Geometry check sheet. Reference: the model listing, model coordinates, mm. Round coordinates to 2 decimals unless told otherwise and drop trailing zeros. Loops run counter-clockwise (first coordinate to the right, second up) from the corner with the lowest first, then second, coordinate; pieces in that order, holes last. Notation, with made-up numbers: (62.25, 22.25) - (82.25, 22.25) arc R15 cw to (82.25, 36.25) - close; hole circle Ø6 at (22, 71). An arc over 180 degrees is marked (long way). Answer as CSV lines item,"result". Start each with the question number.
1) Cross-section at D-D on x = 65. Record the boundary of the cut face in (y, z).
2) Thickness scan on line 1 along X through (y, z) = (0.9, -57); line 2 along X through (y, z) = (2.25, -175); line 3 along X through (y, z) = (1.7, -333). Record the ranges inside material, lowest first.
3) Cross-section at A-A on z = -260.5. Record the boundary of the cut face in (x, y).
4) Depth check by flat-ended pin: P1, Ø2.5, axis at y = 2, z = -341.5, coming from the -X side; P2, Ø10, axis at x = 152, z = -266.5, coming from the -Y side. Enter the tip coordinate at first touch or a pass-through.
5) Cross-section at B-B on x = 34.5. Record the boundary of the cut face in (y, z), and give its area (3 significant figures).
6) Draft check along Z on faces 1 (the cylindrical face through (246.99, 2.46, -2.85)), 2 (the cylindrical face through (247.15, 2.46, -346.99)), 3 (the cylindrical face through (162.63, 2.46, -169.27)). Enter one of: released by +Z, released by -Z, zero draft, split by the parting line, or undercut.
7) Cross-section at C-C on z = -213. Record the boundary of the cut face in (x, y), and give its area (3 significant figures).
from build123d import *

# Parameters (mm, degrees)
SKETCH1_R           = 1.5
SKETCH1_W           = 30
SKETCH1_H           = 5
SKETCH1_W_2         = 5
SKETCH1_H_2         = 50
SKETCH1_R_2         = 3
SKETCH1_R_3         = 4
SKETCH1_W_3         = 60
SKETCH1_R_4         = 6.2
SKETCH1_R_5         = 9.5
SKETCH1_W_4         = 98
SKETCH1_H_3         = 41
SKETCH1_H_4         = 100
BOSS_EXTRUDE1_DEPTH = 5


with BuildPart() as part:
    # Sketch1 → Boss-Extrude1 (new body)
    # profile 1 of 2: a face of its own
    with BuildSketch(Plane(origin=(0, 0, 0), x_dir=(1, 0, 0), z_dir=(0, 1, 0))):
        with BuildLine():
            ThreePointArc((0, 10), (2.928932188, 2.928932188), (10, 0))
            Line((10, 0), (240, 0))
            ThreePointArc((240, 0), (247.071067812, 2.928932188), (250, 10))
            Line((250, 10), (250, 340))
            ThreePointArc((250, 340), (247.071067812, 347.071067812), (240, 350))
            Line((240, 350), (10, 350))
            ThreePointArc((10, 350), (2.928932188, 347.071067812), (0, 340))
            Line((0, 340), (0, 10))
        make_face()
        with Locations(Location((17, 17, 0), (0, 0, 270))):
            Circle(SKETCH1_R, mode=Mode.SUBTRACT)
        with Locations((42, 9.5)):
            Rectangle(SKETCH1_W, SKETCH1_H, mode=Mode.SUBTRACT)
        with Locations((9.5, 52)):
            Rectangle(SKETCH1_W_2, SKETCH1_H_2, mode=Mode.SUBTRACT)
        with Locations(Location((45, 147.266112644, 0), (0, 0, 270))):
            Circle(SKETCH1_R_2, mode=Mode.SUBTRACT)
        with Locations(Location((65, 125, 0), (0, 0, 270))):
            Circle(SKETCH1_R_3, mode=Mode.SUBTRACT)
        with Locations(Location((105, 125, 0), (0, 0, 270))):
            Circle(SKETCH1_R_3, mode=Mode.SUBTRACT)
        with Locations((125, 9.5)):
            Rectangle(SKETCH1_W_3, SKETCH1_H, mode=Mode.SUBTRACT)
        with Locations((208, 9.5)):
            Rectangle(SKETCH1_W, SKETCH1_H, mode=Mode.SUBTRACT)
        with Locations(Location((233, 17, 0), (0, 0, 270))):
            Circle(SKETCH1_R, mode=Mode.SUBTRACT)
        with Locations((240.5, 52)):
            Rectangle(SKETCH1_W_2, SKETCH1_H_2, mode=Mode.SUBTRACT)
        with Locations(Location((145, 125, 0), (0, 0, 270))):
            Circle(SKETCH1_R_3, mode=Mode.SUBTRACT)
        with Locations(Location((185, 125, 0), (0, 0, 270))):
            Circle(SKETCH1_R_3, mode=Mode.SUBTRACT)
        with Locations(Location((205, 147.266112644, 0), (0, 0, 270))):
            Circle(SKETCH1_R_2, mode=Mode.SUBTRACT)
        Polygon((7, 175), (7, 225), (12, 225), (12, 125), (7, 125), align=None, mode=Mode.SUBTRACT)
        with Locations(Location((17, 206, 0), (0, 0, 270))):
            Circle(SKETCH1_R, mode=Mode.SUBTRACT)
        with Locations(Location((45, 202.733887356, 0), (0, 0, 270))):
            Circle(SKETCH1_R_2, mode=Mode.SUBTRACT)
        with Locations(Location((85, 175, 0), (0, 0, 270))):
            Circle(SKETCH1_R_4, mode=Mode.SUBTRACT)
        with Locations(Location((78.5, 225.5, 0), (0, 0, 270))):
            Circle(SKETCH1_R, mode=Mode.SUBTRACT)
        with Locations((9.5, 298)):
            Rectangle(SKETCH1_W_2, SKETCH1_H_2, mode=Mode.SUBTRACT)
        with Locations(Location((17, 333, 0), (0, 0, 270))):
            Circle(SKETCH1_R, mode=Mode.SUBTRACT)
        with Locations((42, 340.5)):
            Rectangle(SKETCH1_W, SKETCH1_H, mode=Mode.SUBTRACT)
        with Locations(Location((78.5, 280.5, 0), (0, 0, 270))):
            Circle(SKETCH1_R, mode=Mode.SUBTRACT)
        with Locations(Location((125, 175, 0), (0, 0, 270))):
            Circle(SKETCH1_R_5, mode=Mode.SUBTRACT)
        with Locations(Location((165, 175, 0), (0, 0, 270))):
            Circle(SKETCH1_R_4, mode=Mode.SUBTRACT)
        with Locations((125, 253)):
            Rectangle(SKETCH1_W_4, SKETCH1_H_3, mode=Mode.SUBTRACT)
        with Locations(Location((171.5, 225.5, 0), (0, 0, 270))):
            Circle(SKETCH1_R, mode=Mode.SUBTRACT)
        with Locations(Location((205, 202.733887356, 0), (0, 0, 270))):
            Circle(SKETCH1_R_2, mode=Mode.SUBTRACT)
        with Locations((240.5, 175)):
            Rectangle(SKETCH1_W_2, SKETCH1_H_4, mode=Mode.SUBTRACT)
        with Locations(Location((233, 206, 0), (0, 0, 270))):
            Circle(SKETCH1_R, mode=Mode.SUBTRACT)
        with Locations(Location((171.5, 280.5, 0), (0, 0, 270))):
            Circle(SKETCH1_R, mode=Mode.SUBTRACT)
        Polygon((95, 343), (125, 343), (155, 343), (155, 338), (95, 338), align=None, mode=Mode.SUBTRACT)
        with Locations((240.5, 298)):
            Rectangle(SKETCH1_W_2, SKETCH1_H_2, mode=Mode.SUBTRACT)
        with Locations((208, 340.5)):
            Rectangle(SKETCH1_W, SKETCH1_H, mode=Mode.SUBTRACT)
        with Locations(Location((233, 333, 0), (0, 0, 270))):
            Circle(SKETCH1_R, mode=Mode.SUBTRACT)
    # profile 2 of 2: a face of its own
    with BuildSketch(Plane(origin=(0, 0, 0), x_dir=(1, 0, 0), z_dir=(0, 1, 0))):
        with BuildLine():
            ThreePointArc((0, 10), (2.928932188, 2.928932188), (10, 0))
            Line((10, 0), (240, 0))
            ThreePointArc((240, 0), (247.071067812, 2.928932188), (250, 10))
            Line((250, 10), (250, 340))
            ThreePointArc((250, 340), (247.071067812, 347.071067812), (240, 350))
            Line((240, 350), (10, 350))
            ThreePointArc((10, 350), (2.928932188, 347.071067812), (0, 340))
            Line((0, 340), (0, 10))
        make_face()
        with Locations(Location((17, 17, 0), (0, 0, 270))):
            Circle(SKETCH1_R, mode=Mode.SUBTRACT)
        with Locations((42, 9.5)):
            Rectangle(SKETCH1_W, SKETCH1_H, mode=Mode.SUBTRACT)
        with Locations((9.5, 52)):
            Rectangle(SKETCH1_W_2, SKETCH1_H_2, mode=Mode.SUBTRACT)
        with Locations(Location((45, 147.266112644, 0), (0, 0, 270))):
            Circle(SKETCH1_R_2, mode=Mode.SUBTRACT)
        with Locations(Location((65, 125, 0), (0, 0, 270))):
            Circle(SKETCH1_R_3, mode=Mode.SUBTRACT)
        with Locations(Location((105, 125, 0), (0, 0, 270))):
            Circle(SKETCH1_R_3, mode=Mode.SUBTRACT)
        with Locations((125, 9.5)):
            Rectangle(SKETCH1_W_3, SKETCH1_H, mode=Mode.SUBTRACT)
        with Locations((208, 9.5)):
            Rectangle(SKETCH1_W, SKETCH1_H, mode=Mode.SUBTRACT)
        with Locations(Location((233, 17, 0), (0, 0, 270))):
            Circle(SKETCH1_R, mode=Mode.SUBTRACT)
        with Locations((240.5, 52)):
            Rectangle(SKETCH1_W_2, SKETCH1_H_2, mode=Mode.SUBTRACT)
        with Locations(Location((145, 125, 0), (0, 0, 270))):
            Circle(SKETCH1_R_3, mode=Mode.SUBTRACT)
        with Locations(Location((185, 125, 0), (0, 0, 270))):
            Circle(SKETCH1_R_3, mode=Mode.SUBTRACT)
        with Locations(Location((205, 147.266112644, 0), (0, 0, 270))):
            Circle(SKETCH1_R_2, mode=Mode.SUBTRACT)
        Polygon((7, 175), (7, 225), (12, 225), (12, 125), (7, 125), align=None, mode=Mode.SUBTRACT)
        with Locations(Location((17, 206, 0), (0, 0, 270))):
            Circle(SKETCH1_R, mode=Mode.SUBTRACT)
        with Locations(Location((45, 202.733887356, 0), (0, 0, 270))):
            Circle(SKETCH1_R_2, mode=Mode.SUBTRACT)
        with Locations(Location((85, 175, 0), (0, 0, 270))):
            Circle(SKETCH1_R_4, mode=Mode.SUBTRACT)
        with Locations(Location((78.5, 225.5, 0), (0, 0, 270))):
            Circle(SKETCH1_R, mode=Mode.SUBTRACT)
        with Locations((9.5, 298)):
            Rectangle(SKETCH1_W_2, SKETCH1_H_2, mode=Mode.SUBTRACT)
        with Locations(Location((17, 333, 0), (0, 0, 270))):
            Circle(SKETCH1_R, mode=Mode.SUBTRACT)
        with Locations((42, 340.5)):
            Rectangle(SKETCH1_W, SKETCH1_H, mode=Mode.SUBTRACT)
        with Locations(Location((78.5, 280.5, 0), (0, 0, 270))):
            Circle(SKETCH1_R, mode=Mode.SUBTRACT)
        with Locations(Location((125, 175, 0), (0, 0, 270))):
            Circle(SKETCH1_R_5, mode=Mode.SUBTRACT)
        with Locations(Location((165, 175, 0), (0, 0, 270))):
            Circle(SKETCH1_R_4, mode=Mode.SUBTRACT)
        with Locations((125, 253)):
            Rectangle(SKETCH1_W_4, SKETCH1_H_3, mode=Mode.SUBTRACT)
        with Locations(Location((171.5, 225.5, 0), (0, 0, 270))):
            Circle(SKETCH1_R, mode=Mode.SUBTRACT)
        with Locations(Location((205, 202.733887356, 0), (0, 0, 270))):
            Circle(SKETCH1_R_2, mode=Mode.SUBTRACT)
        with Locations((240.5, 175)):
            Rectangle(SKETCH1_W_2, SKETCH1_H_4, mode=Mode.SUBTRACT)
        with Locations(Location((233, 206, 0), (0, 0, 270))):
            Circle(SKETCH1_R, mode=Mode.SUBTRACT)
        with Locations(Location((171.5, 280.5, 0), (0, 0, 270))):
            Circle(SKETCH1_R, mode=Mode.SUBTRACT)
        Polygon((95, 343), (125, 343), (155, 343), (155, 338), (95, 338), align=None, mode=Mode.SUBTRACT)
        with Locations((240.5, 298)):
            Rectangle(SKETCH1_W_2, SKETCH1_H_2, mode=Mode.SUBTRACT)
        with Locations((208, 340.5)):
            Rectangle(SKETCH1_W, SKETCH1_H, mode=Mode.SUBTRACT)
        with Locations(Location((233, 333, 0), (0, 0, 270))):
            Circle(SKETCH1_R, mode=Mode.SUBTRACT)
    extrude(amount=BOSS_EXTRUDE1_DEPTH)


solid = part.part
Answer block:
1,outline,"(0, -350) - (5, -350) - (5, -129) - (0, -129) - close; (0, -121) - (5, -121) - (5, 0) - (0, 0) - close"
2,line 1,"x = 0 to 7, 12 to 238, 243 to 250"
2,line 2,"x = 0 to 7, 12 to 78.8, 91.2 to 115.5, 134.5 to 158.8, 171.2 to 238, 243 to 250"
2,line 3,"x = 0 to 15.5, 18.5 to 231.5, 234.5 to 250"
3,outline,"(0, 0) - (76, 0) - (76, 5) - (0, 5) - close; (174, 0) - (250, 0) - (250, 5) - (174, 5) - close"
4,P1,"stops at x = 0"
4,P2,"passes through"
5,outline,"(0, -350) - (5, -350) - (5, -343) - (0, -343) - close; (0, -338) - (5, -338) - (5, -12) - (0, -12) - close; (0, -7) - (5, -7) - (5, 0) - (0, 0) - close"
5,area,"1,700 mm^2"
6,face 1,"released by +Z"
6,face 2,"released by -Z"
6,face 3,"undercut"
7,outline,"(0, 0) - (7, 0) - (7, 5) - (0, 5) - close; (12, 0) - (238, 0) - (238, 5) - (12, 5) - close; (243, 0) - (250, 0) - (250, 5) - (243, 5) - close"
7,area,"1,200 mm^2"
